The model under review builds one solid part; all positions refer to its coordinate system, in mm. Face numbers are marked on the shaded views. Coordinates: 2 decimals unless noted, no trailing zeros. Order: outer loops, then holes, each group sorted by start corner. A loop starts at its lowest first (then second) coordinate and runs counter-clockwise, first axis right, second up. Notation, with made-up numbers: (52, 51) -> (56, 51) arc R29 cw to (56, 79) -> close; hole circle Ø3 at (58, 24). An arc over 180 degrees is marked (long way). Use one line per item in the form item = value.
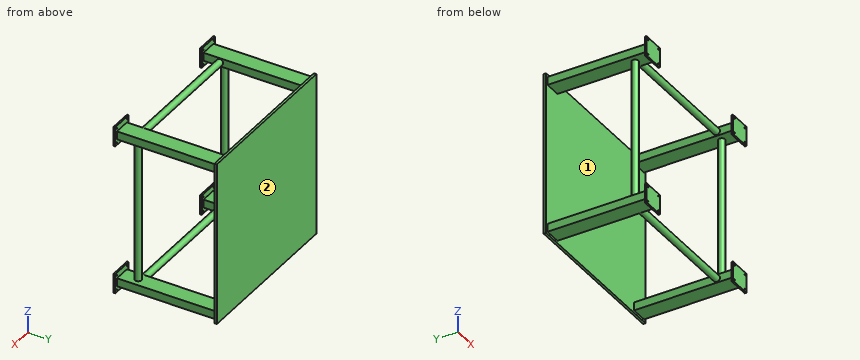
from build123d import *

# Parameters (mm, degrees)
SKETCH1_W               = 1000
SKETCH1_H               = 1000
BOSS_EXTRUDE1_DEPTH     = 15
SKETCH2_W               = 100
SKETCH2_H               = 50
BOSS_EXTRUDE2_DEPTH     = 605
SKETCH3_W               = 135
SKETCH3_H               = 120
BOSS_EXTRUDE3_DEPTH     = 10
SKETCH5_R               = 4
CUT_EXTRUDE1_DEPTH      = 10
MIRROR2_COPY_1_SKETCH_W = 100
MIRROR2_COPY_1_SKETCH_H = 50
MIRROR2_COPY_1_DEPTH    = 605
MIRROR2_COPY_2_SKETCH_W = 135
MIRROR2_COPY_2_SKETCH_H = 120
MIRROR2_COPY_2_DEPTH    = 10
MIRROR2_COPY_3_SKETCH_R = 4
MIRROR2_COPY_3_DEPTH    = 10
SKETCH6_R               = 20
BOSS_EXTRUDE4_DEPTH     = 870
SKETCH7_R               = 20
BOSS_EXTRUDE5_DEPTH     = 770


with BuildPart() as part:
    # Sketch1 → Boss-Extrude1 (new body)
    with BuildSketch(Plane(origin=(0, 0, 0), x_dir=(1, 0, 0), z_dir=(0, 1, 0))):
        Rectangle(SKETCH1_W, SKETCH1_H)
    extrude(amount=BOSS_EXTRUDE1_DEPTH)

    # Sketch2 → Boss-Extrude2 (add)
    with BuildSketch(Plane.XZ):
        with Locations((435, 460)):
            Rectangle(SKETCH2_W, SKETCH2_H)
    boss_extrude2 = extrude(amount=BOSS_EXTRUDE2_DEPTH)

    # Sketch3 → Boss-Extrude3 (add)
    with BuildSketch(Plane.XZ.offset(605)):
        with Locations((435, 460)):
            Rectangle(SKETCH3_W, SKETCH3_H)
    boss_extrude3 = extrude(amount=BOSS_EXTRUDE3_DEPTH)

    # Sketch5 → Cut-Extrude1 (cut)
    with BuildSketch(Plane.XZ.offset(615)):
        with Locations(Location((382.5, 505, 0), (0, 0, 270))):
            Circle(SKETCH5_R)
        with Locations(Location((382.5, 415, 0), (0, 0, 270))):
            Circle(SKETCH5_R)
        with Locations(Location((487.5, 415, 0), (0, 0, 270))):
            Circle(SKETCH5_R)
        with Locations(Location((487.5, 505, 0), (0, 0, 270))):
            Circle(SKETCH5_R)
    cut_extrude1 = extrude(amount=-CUT_EXTRUDE1_DEPTH, mode=Mode.SUBTRACT)

    # Mirror1: Boss-Extrude2, Boss-Extrude3, Cut-Extrude1 across plane
    add(boss_extrude2.mirror(Plane.XY))
    add(boss_extrude3.mirror(Plane.XY))
    add(cut_extrude1.mirror(Plane.XY), mode=Mode.SUBTRACT)

    # Mirror2: Boss-Extrude2, Boss-Extrude3, Cut-Extrude1 across plane
    add(boss_extrude2.mirror(Plane(origin=(0, 0, 0), x_dir=(0, 0, 1), z_dir=(1, 0, 0))))
    add(boss_extrude3.mirror(Plane(origin=(0, 0, 0), x_dir=(0, 0, 1), z_dir=(1, 0, 0))))
    add(cut_extrude1.mirror(Plane(origin=(0, 0, 0), x_dir=(0, 0, 1), z_dir=(1, 0, 0))), mode=Mode.SUBTRACT)

    # Mirror2 copy 1 sketch → Mirror2 copy 1 (add)
    with BuildSketch(Plane(origin=(0, 0, 0), x_dir=(-1, 0, 0), z_dir=(0, -1, 0))):
        with Locations((435, 460)):
            Rectangle(MIRROR2_COPY_1_SKETCH_W, MIRROR2_COPY_1_SKETCH_H)
    extrude(amount=MIRROR2_COPY_1_DEPTH)

    # Mirror2 copy 2 sketch → Mirror2 copy 2 (add)
    with BuildSketch(Plane(origin=(0, -605, 0), x_dir=(-1, 0, 0), z_dir=(0, -1, 0))):
        with Locations((435, 460)):
            Rectangle(MIRROR2_COPY_2_SKETCH_W, MIRROR2_COPY_2_SKETCH_H)
    extrude(amount=MIRROR2_COPY_2_DEPTH)

    # Mirror2 copy 3 sketch → Mirror2 copy 3 (cut)
    with BuildSketch(Plane(origin=(0, -615, 0), x_dir=(-1, 0, 0), z_dir=(0, -1, 0))):
        with Locations(Location((382.5, 505, 0), (0, 0, 270))):
            Circle(MIRROR2_COPY_3_SKETCH_R)
        with Locations(Location((382.5, 415, 0), (0, 0, 270))):
            Circle(MIRROR2_COPY_3_SKETCH_R)
        with Locations(Location((487.5, 415, 0), (0, 0, 270))):
            Circle(MIRROR2_COPY_3_SKETCH_R)
        with Locations(Location((487.5, 505, 0), (0, 0, 270))):
            Circle(MIRROR2_COPY_3_SKETCH_R)
    extrude(amount=-MIRROR2_COPY_3_DEPTH, mode=Mode.SUBTRACT)

    # Sketch6 → Boss-Extrude4 (add)
    with BuildSketch(Plane(origin=(0, 0, 435), x_dir=(-1, 0, 0), z_dir=(0, 0, -1))):
        with Locations(Location((-435, -505, 0), (0, 0, 180))):
            Circle(SKETCH6_R)
    boss_extrude4 = extrude(amount=BOSS_EXTRUDE4_DEPTH)

    # Sketch7 → Boss-Extrude5 (add)
    with BuildSketch(Plane.ZY.offset(-385)):
        with Locations(Location((460, -505, 0), (0, 0, 180))):
            Circle(SKETCH7_R)
    boss_extrude5 = extrude(amount=BOSS_EXTRUDE5_DEPTH)

    # Mirror3: Boss-Extrude5 across plane
    add(boss_extrude5.mirror(Plane.XY))

    # Mirror4: Boss-Extrude4 across plane
    add(boss_extrude4.mirror(Plane(origin=(0, 0, 0), x_dir=(0, 0, 1), z_dir=(1, 0, 0))))


solid = part.part
Item 1: To check wall thickness, follow L1, parallel to X at y = -611.5, z = -505; L2, parallel to Z at x = -487, y = -608; L3, parallel to Y at x = -370.5, z = 10.5. State the ranges of each line that lie inside material, in increasing order. Write a range as from..to.
Results found:
L1 = -502.5..-491.5, -483.5..-386.5, -378.5..-367.5, 367.5..378.5, 386.5..483.5, 491.5..502.5
L2 = -520..-508.97, -501.03..-418.97, -411.03..-400, 400..411.03, 418.97..501.03, 508.97..520
L3 = 0..15
Item 2: Draft analysis for pull direction Y (two halves, no side actions). For the marked faces 1 and 2, state which applies: released by +Y, released by -Y, zero draft, split by the parting line, or undercut.
Results found:
face_1 = undercut
face_2 = released by +Y
Item 3: We need section A-A (y = -332.5). Write out the cut boundary in (x, z).
Results found:
outline = (-485, -485) -> (-385, -485) -> (-385, -435) -> (-485, -435) -> close; (-485, 435) -> (-385, 435) -> (-385, 485) -> (-485, 485) -> close; (385, -485) -> (485, -485) -> (485, -435) -> (385, -435) -> close; (385, 435) -> (485, 435) -> (485, 485) -> (385, 485) -> close
Item 4: We need section B-B (z = 171). Write out the cut boundary in (x, y).
Results found:
outline = (-500, 0) -> (500, 0) -> (500, 15) -> (-500, 15) -> close; circle Ø40 at (-435, -505); circle Ø40 at (435, -505)
Item 5: Clearance check with flat-ended pins moving along their axes: pin 1 (7 mm diameter, centred on x = -487.5, z = -415, fed in from -Y); pin 2 (1 mm diameter, centred on x = -363, y = -514, fed in from -Z); pin 3 (16.5 mm diameter, centred on y = 10.5, z = -111, fed in from -X); pin 4 (7 mm diameter, centred on x = 382.5, z = 505, fed in from -Y). State where each tip first meets the part, or that it passes through.
Results found:
pin_1 = 0
pin_2 = -478.1
pin_3 = -500
pin_4 = through
Item 6: We need section C-C (x = -435). Write out the cut boundary in (y, z).
Results found:
outline = (-615, -520) -> (-605, -520) -> (-605, -485) -> (0, -485) -> (0, -500) -> (15, -500) -> (15, 500) -> (0, 500) -> (0, 485) -> (-605, 485) -> (-605, 520) -> (-615, 520) -> (-615, 400) -> (-605, 400) -> (-605, 435) -> (-525, 435) -> (-525, -435) -> (-605, -435) -> (-605, -400) -> (-615, -400) -> close; hole (-485, -435) -> (0, -435) -> (0, 435) -> (-485, 435) -> close
